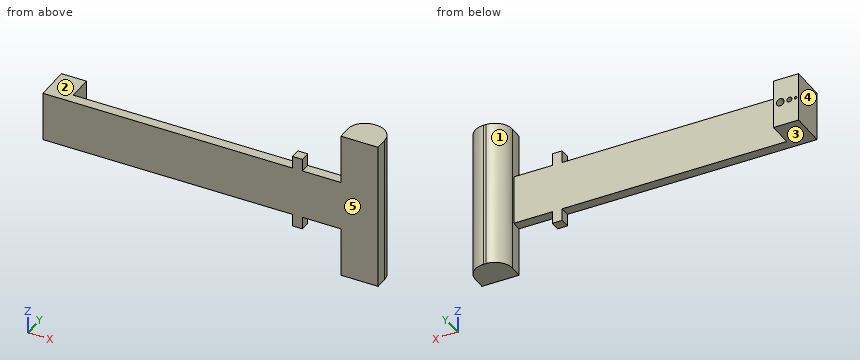
Autodesk Inventor part; units mm, degrees
ref_plane "YZ Plane" through (0, 0, 0) normal (1, 0, 0) x (0, 1, 0)
ref_plane "XZ Plane" through (0, 0, 0) normal (0, 1, 0) x (-1, 0, 0)
ref_plane "XY Plane" through (0, 0, 0) normal (0, 0, 1) x (1, 0, 0)
sketch "rod" plane through (0, 0, 0) normal (0, 1, 0) x (-1, 0, 0)
  line L0 (8.8103, 11.8971) -> (-111.1897, 11.8971)
  line L1 (-111.1897, 11.8971) -> (-111.1897, -8.1029)
  line L2 (-111.1897, -8.1029) -> (8.8103, -8.1029)
  line L3 (8.8103, -8.1029) -> (8.8103, 11.8971)
  point P0 (0, 0)
  dimension "d0" = 20
  dimension "d1" = 120
extrude "Extrusion1" add sketch "rod" along normal blind 4
sketch "Sketch2" plane through (0, 0, 0) normal (0, -1, 0) x (1, 0, 0)
  line L0 (111.1897, 31.8971) -> (126.1897, 31.8971)
  line L1 (126.1897, 31.8971) -> (126.1897, -28.1029)
  line L2 (126.1897, -28.1029) -> (111.1897, -28.1029)
  line L3 (111.1897, -28.1029) -> (111.1897, 31.8971)
  line L4 (111.1897, 11.8971) -> (111.1897, -8.1029)
  line L5 (-8.8103, 11.8971) -> (111.1897, 11.8971)
  point P0 (0, 0)
  dimension "d6" = 15
  dimension "d7" = 60
  dimension "d8" = 20
extrude "Extrusion2" add sketch "Sketch2" against normal blind 12
fillet "Fillet1" radius 7 2 edges at (111.1897, 12, 1.8971) (126.1897, 12, 1.8971)
sketch "Sketch3" plane through (0, 4, 0) normal (0, 1, 0) x (1, 0, 0)
  line L0 (-8.8103, -11.8971) -> (111.1897, -11.8971)
  line L1 (111.1897, 8.1029) -> (-8.8103, 8.1029)
  line L2 (-8.8103, -11.8971) -> (1.2928, -11.8971)
  line L3 (1.2928, -11.8971) -> (1.2928, 8.1029)
  line L4 (1.2928, 8.1029) -> (-8.8103, 8.1029)
  line L5 (-8.8103, 8.1029) -> (-8.8103, -11.8971)
  point P0 (0, 0)
extrude "Extrusion3" add sketch "Sketch3" along normal blind 10
sketch "Sketch4" plane through (0, 14, 0) normal (0, 1, 0) x (1, 0, 0)
  circle A0 centre (-7.6103, -1.8971) radius 0.5166
  circle A1 centre (-5.0911, -1.8971) radius 1.0075
  circle A2 centre (-1.4334, -1.8971) radius 1.5342
  line L0 (-8.8103, -11.8971) -> (1.2928, -11.8971)
  line L1 (-8.8103, 8.1029) -> (-8.8103, -11.8971)
  point P0 (0, 0)
  dimension "d14" = 10
  dimension "d15" = 10
  dimension "d16" = 10
  dimension "d17" = 10.1031
  dimension "d18" = 1.2
extrude "Extrusion4" cut sketch "Sketch4" against normal blind 11.5
sketch "Sketch5" plane through (111.1897, 0, -8.1029) normal (0, 0, -1) x (-1, 0, 0)
  line L0 (0, 4) -> (109.8969, 4)
  line L1 (120, 0) -> (0, 0)
  line L2 (19.4969, 4) -> (15.4969, 4)
  line L3 (15.4969, 4) -> (15.4969, 0)
  line L4 (15.4969, 0) -> (19.4969, 0)
  line L5 (19.4969, 0) -> (19.4969, 4)
  line L6 (109.8969, 4) -> (109.8969, 14)
  point P0 (111.1897, 0)
  dimension "d23" = 4
  dimension "d24" = 90.4
extrude "Extrusion5" add sketch "Sketch5" along normal blind 5
sketch "Sketch6" plane through (-8.8103, 0, 11.8971) normal (0, 0, 1) x (1, 0, 0)
  line L0 (100.5031, 4) -> (10.1031, 4)
  line L1 (100.5031, 0) -> (0, 0)
  line L2 (104.5031, 4) -> (100.5031, 4)
  line L3 (100.5031, 4) -> (100.5031, 0)
  line L4 (100.5031, 0) -> (104.5031, 0)
  line L5 (104.5031, 0) -> (104.5031, 4)
  line L6 (10.1031, 4) -> (10.1031, 14)
  point P0 (8.8103, 0)
  dimension "d27" = 4
  dimension "d28" = 90.4
extrude "Extrusion6" add sketch "Sketch6" along normal blind 5
equation "\"d8\" = 0.25 * d7 + 0.25 * d0"
equation "\"d14\" = 0.5 * d0"
equation "\"d15\" = d14"
equation "\"d16\" = d14"
properties part number "gravity_holder"
Can you work these out from the model? Positions are in its coordinate system, mm. Face numbers are marked on the shaded views. A direction names the side the tool comes from. Round coordinates to 2 decimals unless told otherwise and drop trailing zeros. Order: outer loops, then holes, each group sorted by start corner. A loop starts at its lowest first (then second) coordinate and runs counter-clockwise, first axis right, second up. Notation, with made-up numbers: (57.25, 88) -> (61.25, 88) arc R26 cw to (61.25, 110) -> close; hole circle Ø4 at (14, 53.25). An arc over 180 degrees is marked (long way). Write each question's results on one line, items separated by ' | '. Start each with the question number.
Item 1: Will these pins go through, and if not, where does the flat tip stop? pin 1 (4.5 mm diameter, centred on x = 94, y = 2, fed in from +Z); pin 2 (8 mm diameter, centred on y = 10.5, z = 2.5, fed in from +X); pin 3 (2 mm diameter, centred on x = 106.5, y = 3, fed in from -Z); pin 4 (1.7 mm diameter, centred on x = -7.61, z = 1.9, fed in from -Y).
Item 2: If we section it at C-C, the plane z = -17: Write out the boundary of the cut face in (x, y).
Item 3: If we section it at D-D, the plane x = 82: Write out the boundary of the cut face in (y, z), then the cut area to 3 significant figures.
Item 4: Which directions (+Z, -Z, +X, -X, +Y, -Y) give clear straight access to the entire face, cutting with the end or side of a thin tool? Please do the marked faces 1, 2, 3, 4 and 5.
Item 5: If we section it at A-A, the plane y = 10.25: Write out the boundary of the cut face in (x, z) (1 decimal).
Item 6: If we section it at B-B, the plane z = 15: Write out the boundary of the cut face in (x, y).
Item 7: Please list where these lines run through material, in increasing order: L1, parallel to X at y = 5, z = 9.5; L2, parallel to Y at x = 102.5, z = -1; L3, parallel to Z at x = 3, y = 3.
Results:
1) pin 1: stops at z = 16.9 | pin 2: stops at x = 126.03 | pin 3: stops at z = -8.1 | pin 4: stops at y = 0
2) outline: (111.19, 0) -> (126.19, 0) -> (126.19, 5) arc R7 ccw to (119.19, 12) -> (118.19, 12) arc R7 ccw to (111.19, 5) -> close
3) outline: (0, -8.1) -> (4, -8.1) -> (4, 11.9) -> (0, 11.9) -> close | area: 80.0 mm2
4) face 1: +Z, -Z, +Y | face 2: +Z, -X, +Y, -Y | face 3: -Z, -X, +Y, -Y | face 4: +Z, -Z, -X, +Y, -Y | face 5: +Z, -Z, +X, -X, -Y
5) outline: (-8.8, -8.1) -> (1.3, -8.1) -> (1.3, 11.9) -> (-8.8, 11.9) -> close; (113.6, -28.1) -> (123.8, -28.1) -> (123.8, 31.9) -> (113.6, 31.9) -> close; hole circle Ø1 at (-7.6, 1.9); hole circle Ø2 at (-5.1, 1.9); hole circle Ø3.1 at (-1.4, 1.9)
6) outline: (91.69, 0) -> (95.69, 0) -> (95.69, 4) -> (91.69, 4) -> close; (111.19, 0) -> (126.19, 0) -> (126.19, 5) arc R7 ccw to (119.19, 12) -> (118.19, 12) arc R7 ccw to (111.19, 5) -> close
7) L1: x = -8.81 to 1.29, 111.19 to 126.19 | L2: y = 0 to 4 | L3: z = -8.1 to 11.9
